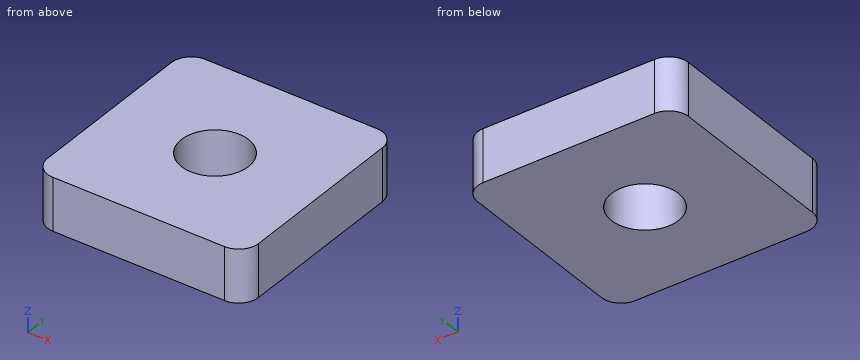
```python
from build123d import *

# Parameters (mm, degrees)
SKETCH_1_W          = 32
SKETCH_1_H          = 32
EXTRUDE_1_DEPTH     = 8
SKETCH_2_R          = 5.1
CUT_EXTRUDE_1_DEPTH = 25
FILLET_1_R          = 3


with BuildPart() as part:
    # Эскиз1 → Бобышка-Вытянуть1 (new body)
    with BuildSketch(Plane.XY):
        Rectangle(SKETCH_1_W, SKETCH_1_H)
    extrude(amount=EXTRUDE_1_DEPTH)

    # Эскиз2 → Вырез-Вытянуть1 (cut, through all)
    with BuildSketch(Plane.XY.offset(8)):
        Circle(SKETCH_2_R)
    extrude(amount=-CUT_EXTRUDE_1_DEPTH, mode=Mode.SUBTRACT)

    # Скругление1
    fillet_1_edges = [part.edges().sort_by_distance(p)[0] for p in [
        (16, -16, 4),
        (-16, -16, 4),
        (-16, 16, 4),
        (16, 16, 4),
    ]]
    fillet(fillet_1_edges, radius=FILLET_1_R)


solid = part.part
```
Could you check a few things on this model? Use its own coordinates, in mm. Round coordinates to 2 decimals unless told otherwise and drop trailing zeros. Loops run counter-clockwise (first coordinate to the right, second up) from the corner with the lowest first, then second, coordinate; pieces in that order, holes last.
Q1. For P1, Ø8, axis at x = 0, y = 0, coming from the -Z side, with a flat end and sliding along its axis, tell me the tip position at first contact or that it passes through.
Q2. I want a section at A-A (x = 0). Write out the boundary of the cut face in (y, z), and give its area (3 significant figures).
Q3. I want a section at B-B (z = 0.75). Write out the boundary of the cut face in (x, y).
Q4. Please list where these lines run through material, in increasing order: L1, parallel to Y at x = 0, z = 3.75; L2, parallel to Y at x = 1.5, z = 1.5; L3, parallel to X at y = -4, z = 4.5.
Answer below:
1. P1: passes through
2. outline: (-16, 0) - (-5.1, 0) - (-5.1, 8) - (-16, 8) - close; (5.1, 0) - (16, 0) - (16, 8) - (5.1, 8) - close
2. area: 174 mm2
3. outline: (-16, -13) arc R3 ccw to (-13, -16) - (13, -16) arc R3 ccw to (16, -13) - (16, 13) arc R3 ccw to (13, 16) - (-13, 16) arc R3 ccw to (-16, 13) - close; hole circle Ø10.2 at (0, 0)
4. L1: y = -16 to -5.1, 5.1 to 16
4. L2: y = -16 to -4.87, 4.87 to 16
4. L3: x = -16 to -3.16, 3.16 to 16
